Answer from the drawing. Dimensions are ordinates in mm from the lowest x, y and z of the part. Coordinates: 2 decimals unless noted, no trailing zeros. Order: outer loops, then holes, each group sorted by start corner. A loop starts at its lowest first (then second) coordinate and runs counter-clockwise, first axis right, second up. Notation, with made-up numbers: (63, 0.5) - (90, 0.5) arc R21 cw to (90, 5.5) - close; hole circle Ø1 at (45.25, 6). An arc over 180 degrees is marked (long way). Use a Markdown table: item, result. Add a question column.
Item 1: The part is cut by section D-D, the plane y = 23.5. Give the vertices of the cut face in (x, z).
Item 2: A flat-ended cylindrical pin translates along its axis: P1, Ø2.5, axis at x = 5, y = 17, coming from the +Z side. Find the tip coordinate at first contact, or state that the pin passes through.
Item 3: Find the intervals of material crossed by line 1 along Y through (x, z) = (24.5, 0.1) (1 decimal); line 2 along Y through (x, z) = (16.5, 0.15) (1 decimal); line 3 along X through (y, z) = (26.5, 0.65), in increasing order.
Item 4: The part is cut by section A-A, the plane x = 17. Give the vertices of the cut face in (y, z), then the cut area to 3 significant figures.
Item 5: The part is cut by section C-C, the plane x = 5. Give the vertices of the cut face in (y, z).
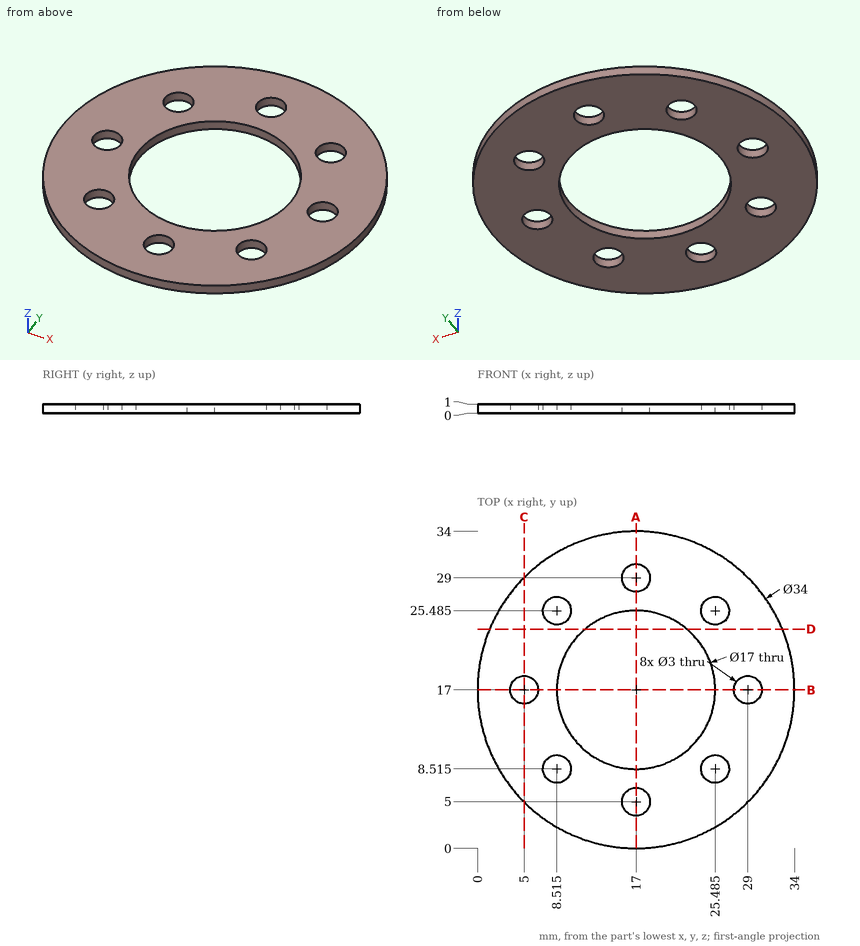
Solution:
| question | item | result |
|---|---|---|
| 1 | outline | (1.29, 0) - (11.52, 0) - (11.52, 1) - (1.29, 1) - close; (22.48, 0) - (32.71, 0) - (32.71, 1) - (22.48, 1) - close |
| 2 | P1 | passes through |
| 3 | line 1 | y = 1.7 to 7.4, 9.6 to 13, 21 to 24.4, 26.6 to 32.3 |
| 3 | line 2 | y = 0 to 3.6, 6.4 to 8.5, 25.5 to 27.6, 30.4 to 34 |
| 3 | line 3 | x = 2.9 to 7.41, 9.62 to 24.38, 26.59 to 31.1 |
| 4 | outline | (0, 0) - (3.5, 0) - (3.5, 1) - (0, 1) - close; (6.5, 0) - (8.5, 0) - (8.5, 1) - (6.5, 1) - close; (25.5, 0) - (27.5, 0) - (27.5, 1) - (25.5, 1) - close; (30.5, 0) - (34, 0) - (34, 1) - (30.5, 1) - close |
| 4 | area | 11.0 mm2 |
| 5 | outline | (4.96, 0) - (15.5, 0) - (15.5, 1) - (4.96, 1) - close; (18.5, 0) - (29.04, 0) - (29.04, 1) - (18.5, 1) - close |
